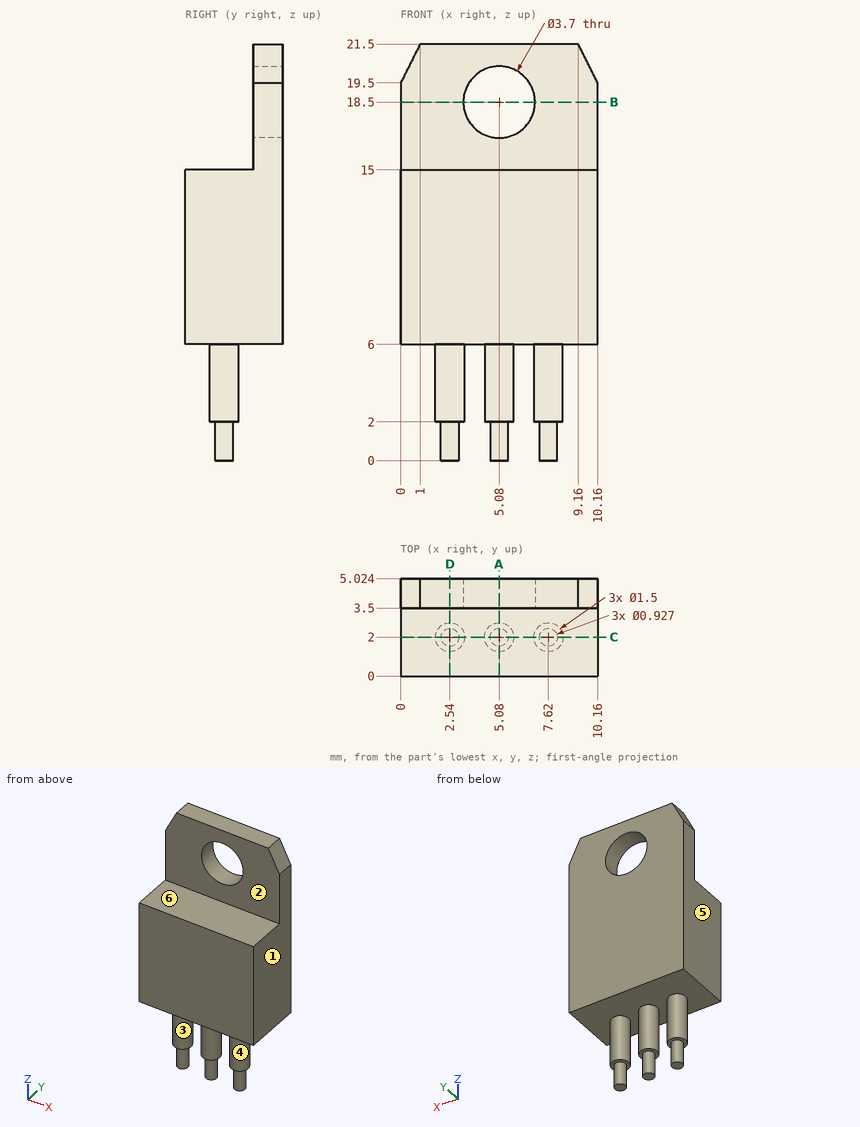
Job drawing, mm, ordinate dimensions from the low corner. One solid piece. A direction names the side the tool comes from. Coordinates: 2 decimals unless noted, no trailing zeros. Order: outer loops, then holes, each group sorted by start corner. A loop starts at its lowest first (then second) coordinate and runs counter-clockwise, first axis right, second up. Notation, with made-up numbers: M 18,75.5 L 32,75.5 A18 ccw 32,94.5 Z; hole C -21,-20.5 d2. An arc over 180 degrees is marked long. One line per question, with ' | ' between items.
Q1. Slice it at D-D (x = 2.54). Give the cut face in (y, z).
A:
outline: M 0,6 L 1.25,6 L 1.25,2 L 1.54,2 L 1.54,0 L 2.46,0 L 2.46,2 L 2.75,2 L 2.75,6 L 5.02,6 L 5.02,21.5 L 3.5,21.5 L 3.5,15 L 0,15 Z
Q2. Pin check, flat tips, straight feed: P1, Ø3, axis at x = 5, z = 17.5, coming from the -Y side; P2, Ø3, axis at x = 6.5, y = 1.5, coming from the +Z side. Stop position of each tip, or through.
A:
P1: stops at y = 3.5 | P2: stops at z = 15
Q3. Slice it at B-B (z = 18.5). Give the cut face in (x, y).
A:
outline: M 0,3.5 L 3.23,3.5 L 3.23,5.02 L 0,5.02 Z; M 6.93,3.5 L 10.16,3.5 L 10.16,5.02 L 6.93,5.02 Z
Q4. Slice it at A-A (x = 5.08). Give the cut face in (y, z).
A:
outline: M 0,6 L 1.25,6 L 1.25,2 L 1.54,2 L 1.54,0 L 2.46,0 L 2.46,2 L 2.75,2 L 2.75,6 L 5.02,6 L 5.02,16.65 L 3.5,16.65 L 3.5,15 L 0,15 Z; M 3.5,20.35 L 5.02,20.35 L 5.02,21.5 L 3.5,21.5 Z
Q5. Drill centre lines: line 1 (Z direction, x = 5.08, y = 4.05); line 2 (X direction, y = 4.05, z = 18.5); line 3 (Z direction, x = 9.25, y = 2.45). Where is each one in solid material? Low to high.
A:
line 1: z = 6 to 16.65, 20.35 to 21.5 | line 2: x = 0 to 3.23, 6.93 to 10.16 | line 3: z = 6 to 15
Q6. 3-axis set-ups, long thin cutter, end or side, ignore diameter. For the marked faces 1, 2 and 3: which of +Z, -Z, +X, -X, +Y, -Y reach the whole face in a straight line?
A:
face 1: +Z, -Z, +X, +Y, -Y | face 2: +Z, +X, -X, -Y | face 3: -Z
Q7. Two-plate mould, pull along X, no slides. Class the marked faces 4, 5 and 6: +X half, -X half, draft (parallel to the pull), parting line (faces both ways), or undercut.
A:
face 4: undercut | face 5: -X half | face 6: draft
Q8. Slice it at C-C (y = 2). Give the cut face in (x, z).
A:
outline: M 0,6 L 1.79,6 L 1.79,2 L 2.08,2 L 2.08,0 L 3,0 L 3,2 L 3.29,2 L 3.29,6 L 4.33,6 L 4.33,2 L 4.62,2 L 4.62,0 L 5.54,0 L 5.54,2 L 5.83,2 L 5.83,6 L 6.87,6 L 6.87,2 L 7.16,2 L 7.16,0 L 8.08,0 L 8.08,2 L 8.37,2 L 8.37,6 L 10.16,6 L 10.16,15 L 0,15 Z
